The listing builds one solid part. Answer for the finished solid, in the listing's coordinates (mm). A direction names the side the tool comes from. Give positions to 0.01 mm unless a question says otherwise; leave off trailing zeros. Write each loop counter-clockwise with the first axis right and the second up, starting at its lowest first coordinate (ties: lowest second). Pieces come first, ordered by that corner, then holes.
```python
from build123d import *

# Parameters (mm, degrees)
F0_W           = 31.0422331095
F0_H           = 79.8228383064
F1_DEPTH       = 101.6
F3_D           = 6.35
F5_D           = 7.493
F5_DEPTH       = 12.7
F5_CBORE_D     = 8.89
F5_CBORE_DEPTH = 6.35
F5_TIP         = 2.2511243092
F6_W           = 47.3317652941
F6_H           = 33.903124404
F7_DEPTH       = 25.4
F8_W           = 6.2107620761
F8_H           = 16.3113800809
F8_H_2         = 9.3631437048
F9_DEPTH       = 101.6


with BuildPart() as f1:
    # F0 (on Top) → F1 (new body)
    with BuildSketch(Plane.XY):
        Rectangle(F0_W, F0_H)
    extrude(amount=F1_DEPTH)

    # F3 (through all)
    with Locations(Plane(origin=(-15.5211165547, 0, 0), x_dir=(0, -1, 0), z_dir=(-1, 0, 0))):
        with Locations((0, 14.7344674915)):
            Hole(F3_D / 2)

    # F5
    with Locations(Plane(origin=(-15.5211165547, 0, 0), x_dir=(0, -1, 0), z_dir=(-1, 0, 0))):
        with Locations((0, 14.7344674915)):
            CounterBoreHole(F5_D / 2, F5_CBORE_D / 2, F5_CBORE_DEPTH, depth=F5_DEPTH)
            with Locations((0, 0, -(F5_DEPTH + F5_TIP / 2))):  # 118° drill point
                Cone(0, F5_D / 2, F5_TIP, mode=Mode.SUBTRACT)

    # F6 (on face) → F7 (join)
    with BuildSketch(Plane(origin=(-15.5211165547, 0, 0), x_dir=(0, -1, 0), z_dir=(-1, 0, 0))):
        with Locations((-17.0762408525, 84.648437798)):
            Rectangle(F6_W, F6_H)
    extrude(amount=-F7_DEPTH)

    # F8 (on face) → F9 (join)
    with BuildSketch(Plane.XY.offset(101.6)):
        with Locations((-3.105381038, -17.5188337453)):
            Rectangle(F8_W, F8_H)
        Polygon((-6.8292533979, 9.3631437048), (-6.8292533979, -9.3631437048), (-6.2107620761, -9.3631437048), (-6.2107620761, 0), (0, 0), (0, -9.3631437048), (6.8292533979, -9.3631437048), (6.8292533979, 9.3631437048), align=None)
        with Locations((-3.105381038, -4.6815718524)):
            Rectangle(F8_W, F8_H_2)
    extrude(amount=F9_DEPTH)


solid = f1.part
```
Item 1: A cutting plane is placed at C-C, the plane x = 5. Give the vertices of the cut face in (y, z) (3 decimals).
Conclusion:
outline: (-39.911, 0) - (39.911, 0) - (39.911, 67.697) - (40.742, 67.697) - (40.742, 101.6) - (9.363, 101.6) - (9.363, 203.2) - (-9.363, 203.2) - (-9.363, 101.6) - (-39.911, 101.6) - close; hole circle Ø6.35 at (0, 14.734)
Item 2: Which of the six approach directions +Z, -Z, +X, -X, +Y, -Y give full straight-line access (tool end or side, diameter ignored) to faces 5 (the face through (-6.211, -18, 152)), 6 (the face through (0, 9.363, 152)), 7 (the face through (-6.829, 0, 152)), 8 (the face through (-12.39, 0.58, 19.14)), 9 (the face through (0, -18, 152))?
Conclusion:
face 5: +Z, -X, -Y
face 6: +Z, +X, -X, +Y
face 7: +Z, -X, +Y, -Y
face 8: -X
face 9: +Z, +X, -Y
Item 3: A cutting plane is placed at D-D, the plane y = -15. Give the vertices of the cut face in (x, z), plus the area to 3 significant figures.
Conclusion:
outline: (-15.52, 0) - (15.52, 0) - (15.52, 101.6) - (0, 101.6) - (0, 203.2) - (-6.21, 203.2) - (-6.21, 101.6) - (-15.52, 101.6) - close
area: 3,780 mm2
Item 4: Consider probe 1 along Z at (x, y) = (-7.5, 0); probe 2 along Z at (x, y) = (-3, 0); probe 3 along Z at (x, y) = (1.5, -15). Determine where each line is inside the solid, lowest interval first.
Conclusion:
probe 1: z = 0 to 10.99, 18.48 to 101.6
probe 2: z = 0 to 10.99, 18.48 to 203.2
probe 3: z = 0 to 101.6
Item 5: A cutting plane is placed at B-B, the plane z = 150. Give the vertices of the cut face in (x, y), plus the area to 3 significant figures.
Conclusion:
outline: (-6.83, -9.36) - (-6.21, -9.36) - (-6.21, -25.67) - (0, -25.67) - (0, -9.36) - (6.83, -9.36) - (6.83, 9.36) - (-6.83, 9.36) - close
area: 357 mm2
Item 6: A cutting plane is placed at A-A, the plane y = 0. Give the vertices of the cut face in (x, z), plus the area to 3 significant figures.
Conclusion:
outline: (-15.52, 0) - (15.52, 0) - (15.52, 11.56) - (-2.48, 11.56) - (-2.82, 10.99) - (-9.17, 10.99) - (-9.17, 10.29) - (-15.52, 10.29) - close; (-15.52, 19.18) - (-9.17, 19.18) - (-9.17, 18.48) - (-2.82, 18.48) - (-2.48, 17.91) - (15.52, 17.91) - (15.52, 101.6) - (6.83, 101.6) - (6.83, 203.2) - (-6.83, 203.2) - (-6.83, 101.6) - (-15.52, 101.6) - close
area: 4,320 mm2
Item 7: Each of these flat-tipped pins is pushed along its axis until it touches: P1, Ø0.9, axis at y = 40.5, z = 89, coming from the +X side; P2, Ø1, axis at x = 2.5, z = 21.5, coming from the +Y side; P3, Ø0.5, axis at x = -6.5, z = 132.5, coming from the -Y side. Where does it stop, or does it pass through?
Conclusion:
P1: stops at x = 9.88
P2: stops at y = 39.91
P3: stops at y = -9.36
Item 8: Determine the mould class of faces 1 (the face through (-5.952, -0.812, 11.077)), 2 (the face through (-2, -4, 203.2)), 3 (the face through (0, 1, 0)), 4 (the face through (0, -39.911, 50)) for opening direction Z: pulls with the +Z half, pulls with the -Z half, needs draft (parallel to the pull), parting line crosses it, or undercut.
Conclusion:
face 1: undercut
face 2: pulls with the +Z half
face 3: pulls with the -Z half
face 4: needs draft
